Could you check a few things on this drawing? It's one solid part, dimensions in mm from its lowest x, y, z. A direction names the side the tool comes from. Give positions to 0.01 mm unless a question says otherwise; leave off trailing zeros. Order: outer loops, then holes, each group sorted by start corner. A loop starts at its lowest first (then second) coordinate and runs counter-clockwise, first axis right, second up.
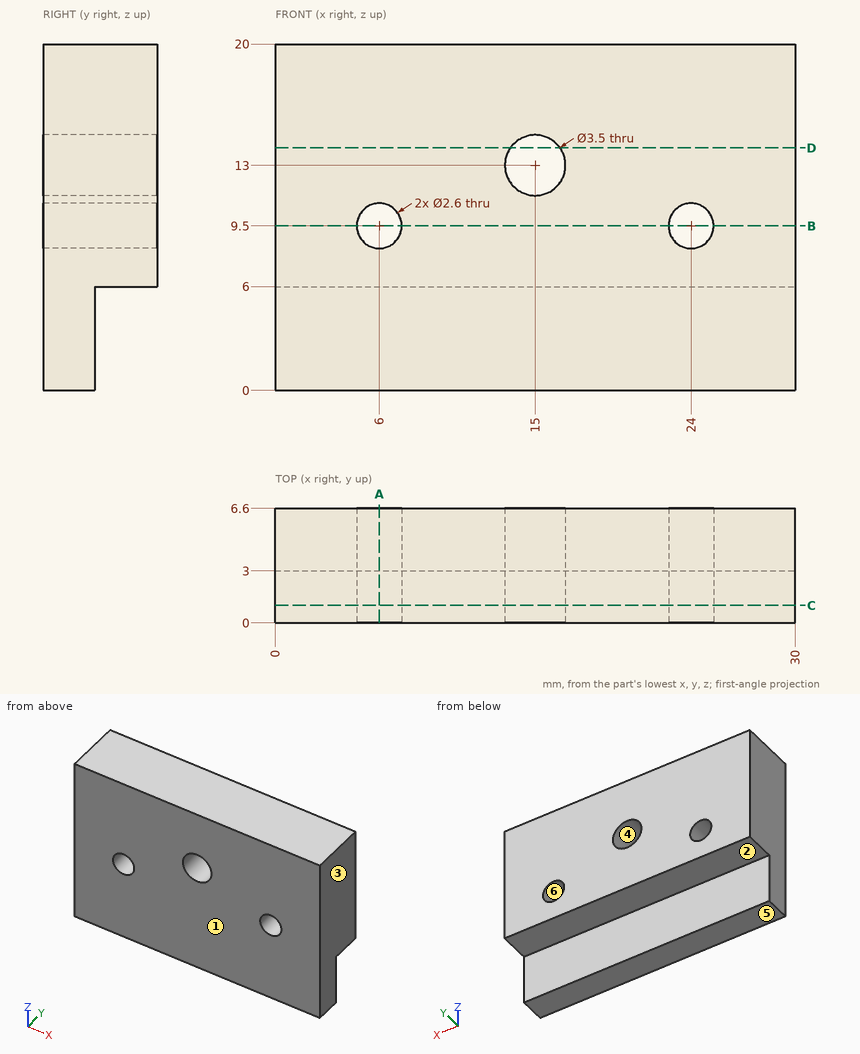
Item 1: Imagine slicing it at B-B on z = 9.5. List the corners of the cut face in (x, y) for me.
Findings:
outline: (0, 0) - (4.7, 0) - (4.7, 6.6) - (0, 6.6) - close; (7.3, 0) - (22.7, 0) - (22.7, 6.6) - (7.3, 6.6) - close; (25.3, 0) - (30, 0) - (30, 6.6) - (25.3, 6.6) - close
Item 2: For the marked faces 1 and 2, which set-ups out of +Z, -Z, +X, -X, +Y, -Y let a thin tool reach every point of the face, with its end or its side?
Findings:
face 1: +Z, -Z, +X, -X, -Y
face 2: -Z, +X, -X, +Y
Item 3: Please list where these lines run through material, in increasing order: line 1 along X through (y, z) = (4.5, 9.5); line 2 along Z through (x, y) = (24, 3.25); line 3 along Z through (x, y) = (24, 2.75).
Findings:
line 1: x = 0 to 4.7, 7.3 to 22.7, 25.3 to 30
line 2: z = 6 to 8.2, 10.8 to 20
line 3: z = 0 to 8.2, 10.8 to 20
Item 4: Imagine slicing it at C-C on y = 1. List the corners of the cut face in (x, z) for me, then the cut area to 3 significant figures.
Findings:
outline: (0, 0) - (30, 0) - (30, 20) - (0, 20) - close; hole circle Ø2.6 at (6, 9.5); hole circle Ø3.5 at (15, 13); hole circle Ø2.6 at (24, 9.5)
area: 580 mm2
Item 5: We'd pull the mould along Z, two halves only. Please class the marked faces 3, 4, 5 and 6: +Z half, -Z half, draft (parallel to the pull), parting line (faces both ways), or undercut.
Findings:
face 3: draft
face 4: undercut
face 5: -Z half
face 6: undercut
Item 6: Imagine slicing it at A-A on x = 6. List the corners of the cut face in (y, z) for me.
Findings:
outline: (0, 0) - (3, 0) - (3, 6) - (6.6, 6) - (6.6, 8.2) - (0, 8.2) - close; (0, 10.8) - (6.6, 10.8) - (6.6, 20) - (0, 20) - close
Item 7: For pin 1 (6.5 mm diameter, centred on x = 13, z = 2.5, fed in from +Y), with a flat end and sliding along its axis, tell me the tip position at first contact or that it passes through.
Findings:
pin 1: stops at y = 3
Item 8: Imagine slicing it at D-D on z = 14. List the corners of the cut face in (x, y) for me, then the cut area to 3 significant figures.
Findings:
outline: (0, 0) - (13.56, 0) - (13.56, 6.6) - (0, 6.6) - close; (16.44, 0) - (30, 0) - (30, 6.6) - (16.44, 6.6) - close
area: 179 mm2
